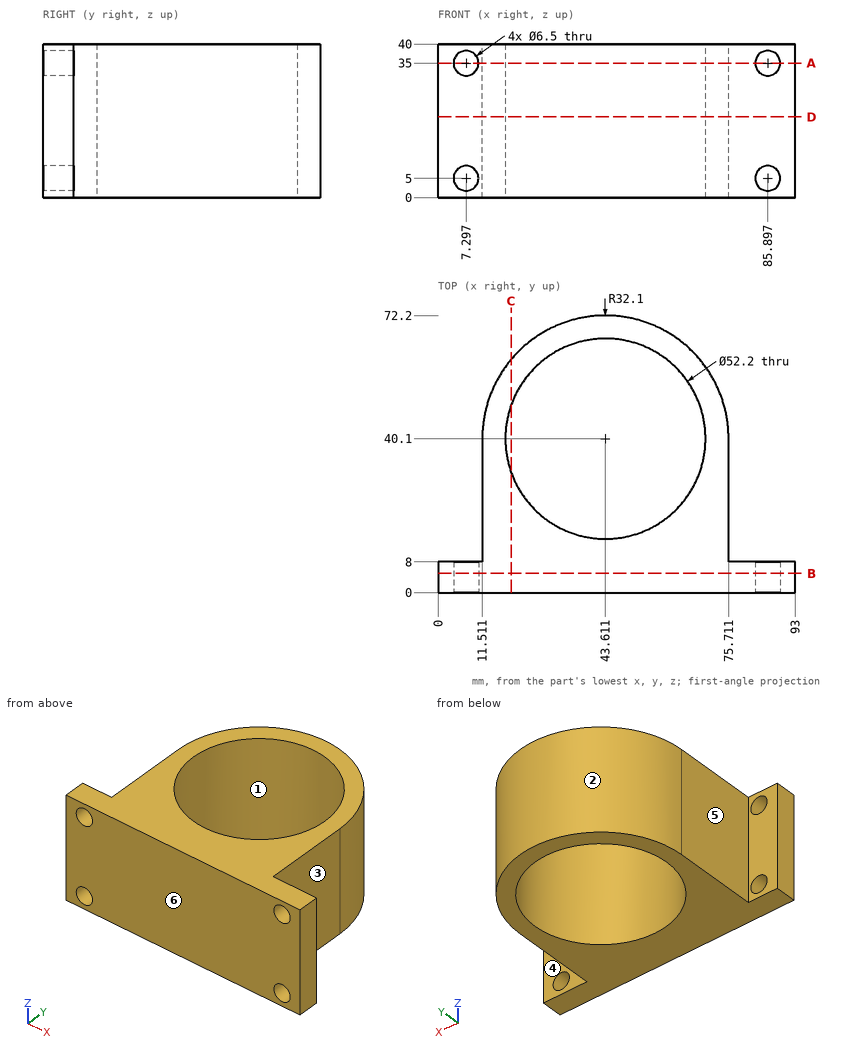
Verification items for this drawing (mm, ordinates from the low corner). A direction names the side the tool comes from. Give positions to 0.01 mm unless a question says otherwise; leave off trailing zeros. Loops run counter-clockwise (first coordinate to the right, second up) from the corner with the lowest first, then second, coordinate; pieces in that order, holes last. Notation, with made-up numbers: M 7.25,87 L 61.25,87 A17 ccw 61.25,101 Z; hole C 14.25,6 d9. An arc over 180 degrees is marked long. Write item = value, one per line. Start each with the question number.
1. Thickness scan on probe 1 along X at (y, z) = (4.5, 35); probe 2 along Y at (x, z) = (5.5, 29.5); probe 3 along X at (y, z) = (53.5, 14) (1 decimal). Record the ranges inside material, lowest first.
2. Section check A-A, the plane z = 35. Enter the section's corners in (x, y), plus the area to 3 significant figures.
3. Section check D-D, the plane z = 21. Enter the section's corners in (x, y), plus the area to 3 significant figures.
4. Section check B-B, the plane y = 5. Enter the section's corners in (x, z).
5. Go/stop test with flat-tipped pins: P1, Ø6, axis at y = 43.5, z = 7.5, coming from the +X side; P2, Ø2, axis at x = 71, z = 27, coming from the +Y side (1 decimal); P3, Ø6, axis at x = 85.9, z = 5, coming from the +Y side; P4, Ø9, axis at x = 4, z = 26.5, coming from the +Y side. Record where each tip stops, or that it passes through.
6. Section check C-C, the plane x = 19. Enter the section's corners in (y, z), plus the area to 3 significant figures.
7. Tool access check on the marked faces 5 and 6. Record the directions out of +Z, -Z, +X, -X, +Y, -Y that give a thin tool (end or side, any length) a straight path to the whole face; none if there is none.
8. Draft check along X on the marked faces 1, 2, 3 and 4. Enter one of: +X half, -X half, draft (parallel to the pull), parting line (faces both ways), or undercut.
Values follow:
q1.probe_1 = 0 to 4.05, 10.55 to 82.65, 89.15 to 93
q1.probe_2 = 0 to 8
q1.probe_3 = 14.4 to 21.2, 66 to 72.8
q2.outline = M 0,0 L 4.05,0 L 4.05,8 L 0,8 Z; M 10.55,0 L 82.65,0 L 82.65,8 L 75.71,8 L 75.71,40.1 A32.1 ccw 11.51,40.1 L 11.51,8 L 10.55,8 Z; M 89.15,0 L 93,0 L 93,8 L 89.15,8 Z; hole C 43.61,40.1 d52.2
q2.area = 2,180 mm^2
q3.outline = M 0,0 L 93,0 L 93,8 L 75.71,8 L 75.71,40.1 A32.1 ccw 11.51,40.1 L 11.51,8 L 0,8 Z; hole C 43.61,40.1 d52.2
q3.area = 2,280 mm^2
q4.outline = M 0,0 L 93,0 L 93,40 L 0,40 Z; hole C 7.3,5 d6.5; hole C 7.3,35 d6.5; hole C 85.9,5 d6.5; hole C 85.9,35 d6.5
q5.P1 = 75.71
q5.P2 = 58.4
q5.P3 = through
q5.P4 = 8
q6.outline = M 0,0 L 31.41,0 L 31.41,40 L 0,40 Z; M 48.79,0 L 60.71,0 L 60.71,40 L 48.79,40 Z
q6.area = 1,730 mm^2
q7.face_5 = +Z, -Z, -X, +Y
q7.face_6 = +Z, -Z, +X, -X, -Y
q8.face_1 = undercut
q8.face_2 = parting line
q8.face_3 = +X half
q8.face_4 = draft
